Autodesk Inventor part; units mm, degrees
ref_plane "YZ Plane" through (0, 0, 0) normal (1, 0, 0) x (0, 1, 0)
ref_plane "XZ Plane" through (0, 0, 0) normal (0, 1, 0) x (-1, 0, 0)
ref_plane "XY Plane" through (0, 0, 0) normal (0, 0, 1) x (1, 0, 0)
sketch "Sketch1" plane through (0, 0, 0) normal (0, 1, 0) x (-1, 0, 0)
  circle A0 centre (0, 0) radius 56.769
  circle A1 centre (0, 0) radius 46.0756
  circle A2 centre (0, 0) radius 31.75
  dimension "d0" = 113.538
  dimension "d1" = 92.1512
  dimension "d2" = 63.5
extrude "Extrusion1" add sketch "Sketch1" along normal blind 17.272 contours A0 | A1 | A2
sketch "Sketch2" plane through (0, 17.272, 0) normal (0, 1, 0) x (1, 0, 0)
  circle A0 centre (0, 0) radius 46.0756
  circle A1 centre (-46.0756, 0) radius 4.0894
  dimension "d5" = 92.1512
  dimension "d6" = 8.1788
hole "Hole1" at (-46.0756, 17.272, 0) direction (0, -1, 0) diameter 8.4328 end through all
pattern_circular "Circular Pattern1" count 8 over 360 about axis through (0, 0, 0) along (0, 1, 0) of "Hole1"
sketch "Sketch4" plane through (0, 17.272, 0) normal (0, 1, 0) x (1, 0, 0)
  circle A0 centre (0, 0) radius 14.7993
hole "Hole2" at (0, 17.272, 0) direction (0, -1, 0) diameter 63.5 end through all
sketch "Sketch6" plane through (0, 0, 0) normal (0, 1, 0) x (-1, 0, 0)
  circle A0 centre (0, 0) radius 31.75
  circle A1 centre (0, 0) radius 19.05
extrude "Extrusion3" add sketch "Sketch6" along normal blind 17.272
sketch "Sketch7" plane through (0, 17.272, 0) normal (0, 1, 0) x (1, 0, 0)
  circle A0 centre (0, 0) radius 34.29
  circle A1 centre (0, 0) radius 31.75
  circle A2 centre (0, 0) radius 25.4
  circle A3 centre (0, 0) radius 27.94
  dimension "d35" = 68.58
  dimension "d36" = 63.5
  dimension "d37" = 50.8
  dimension "d38" = 55.88
extrude "Extrusion4" cut sketch "Sketch7" against normal blind 1.27 contours A0
sketch "Sketch9" plane through (0, 17.272, 0) normal (0, 1, 0) x (1, 0, 0)
  circle A0 centre (0, 0) radius 27.94
  circle A1 centre (0, 0) radius 31.75
  dimension "d45" = 55.88
  dimension "d46" = 63.5
extrude "Extrusion6" cut sketch "Sketch9" against normal blind 2.54
chamfer "Chamfer1" distance 0.254 angle 45 1 edges at (-46.0756, 17.272, -4.2164)
chamfer "Chamfer2" distance 0.254 angle 45 1 edges at (-46.0756, 0, -4.2164)
chamfer "Chamfer3" distance 0.762 angle 45 2 edges at (56.769, 17.272, 0) (56.769, 0, 0)
sketch "Sketch10" plane through (0, 17.272, 0) normal (0, 1, 0) x (1, 0, 0)
  circle A0 centre (32.5804, 32.5804) radius 4.2164
  circle A1 centre (46.0756, 0) radius 4.2164
  line L0 (32.5804, 32.5804) -> (46.0756, 0)
  line L1 (46.0756, 0) -> (39.328, 16.2902)
  circle A2 centre (-46.0756, 0) radius 4.4704
  circle A3 centre (-32.5804, -32.5804) radius 4.2164
  line L2 (-46.0756, 0) -> (-32.5804, -32.5804)
  line L3 (39.328, 16.2902) -> (-39.328, -16.2902)
  line L4 (-39.328, -16.2902) -> (52.9444, 21.9303)
  line L5 (-39.328, -16.2902) -> (60.5469, -16.2902) construction
  line L6 (52.9444, 21.9303) -> (-52.9809, -21.9454)
  line L7 (39.328, 16.2902) -> (39.6342, 15.551)
  line L8 (39.6342, 15.551) -> (39.0218, 17.0294)
  line L9 (39.0218, 17.0294) -> (52.0886, 22.4418)
  line L10 (39.0218, 17.0294) -> (53.1652, 17.0294) construction
  line L11 (52.0886, 22.4418) -> (31.2876, 13.8258)
  line L12 (39.6342, 15.551) -> (52.7487, 20.9832)
  circle A4 centre (0, 0) radius 56.769
  line L13 (39.6342, 15.551) -> (53.8292, 15.551) construction
  line L14 (52.7487, 20.9832) -> (52.7487, 20.9832)
  line L15 (52.7487, 20.9832) -> (31.9774, 12.3794)
  circle A5 centre (0, 0) radius 34.29
  line L16 (31.2876, 13.8258) -> (52.0886, 22.4418)
  line L17 (52.0886, 22.4418) -> (52.7487, 20.9832)
  line L18 (52.0886, 22.4418) -> (31.2876, 13.8258)
  point P0 (31.365, 13.8578)
  dimension "d58" = 22.5
  dimension "d59" = 0.8001
  dimension "d60" = 1.6002
  dimension "d61" = 22.5
  dimension "d62" = 22.5
extrude "Extrusion7" cut sketch "Sketch10" against normal blind 1.016 contours L9 L17 L4 L0 | L0 L3 A5 L11 | L4 L17 L12 L0 | L0 L15 A5 L3
sketch "Sketch11" plane through (0, 17.272, 0) normal (0, 1, 0) x (1, 0, 0)
  line L0 (31.365, 13.8578) -> (51.4323, 22.17)
  line L1 (52.0446, 20.6916) -> (31.9774, 12.3794)
  line L2 (51.4323, 22.17) -> (31.365, 13.8578)
  line L3 (31.365, 13.8578) -> (-52.6609, -20.9468)
  line L4 (52.0446, 20.6916) -> (31.9774, 12.3794)
  circle A0 centre (0, 0) radius 56.769
  line L5 (-52.1363, -22.4616) -> (31.9774, 12.3794)
  line L6 (-52.1363, -22.4616) -> (-52.6609, -20.9468)
  arc A1 (31.365, 13.8578) -> (31.9774, 12.3794) centre (0, 0) ccw
  circle A2 centre (0, 0) radius 34.29
  line L7 (-31.365, -13.8578) -> (-31.9774, -12.3794)
  point P0 (-31.365, -13.8578)
extrude "Extrusion8" cut sketch "Sketch11" against normal blind 1.016 contours A1 L5 L6 L3
sketch "Sketch13" plane through (0, 0, 0) normal (0, -1, 0) x (1, 0, 0)
  circle A0 centre (0, 0) radius 27.94
  circle A1 centre (0, 0) radius 31.75
  circle A2 centre (0, 0) radius 34.29
extrude "Extrusion9" cut sketch "Sketch13" against normal blind 2.54 contours A1
extrude "Extrusion10" cut sketch "Sketch13" against normal blind 1.27 contours A2
sketch "Sketch14" plane through (0, 0, 0) normal (0, -1, 0) x (1, 0, 0)
  line L0 (31.365, -13.8578) -> (52.0886, -22.4418)
  line L1 (52.7487, -20.9832) -> (31.9774, -12.3794)
  line L2 (-52.6609, 20.9468) -> (-31.9774, 12.3794)
  line L3 (-31.365, 13.8578) -> (-52.1363, 22.4616)
  line L4 (51.4323, -22.17) -> (52.0886, -22.4418)
  line L5 (52.0886, -22.4418) -> (31.365, -13.8578)
  arc A0 (52.7487, -20.9832) -> (-52.1363, 22.4616) centre (0, 0) ccw
  line L6 (31.9774, -12.3794) -> (52.7487, -20.9832)
  line L7 (52.7487, -20.9832) -> (52.0886, -22.4418)
  circle A1 centre (0, 0) radius 34.29
  line L8 (-31.9774, 12.3794) -> (-31.365, 13.8578)
  circle A2 centre (0, 0) radius 56.769
  line L9 (-52.1363, 22.4616) -> (-52.6609, 20.9468)
extrude "Extrusion11" cut sketch "Sketch14" against normal blind 1.016 contours A1 L1 L7 L0
extrude "Extrusion12" cut sketch "Sketch14" against normal blind 1.016 contours L2 L9 L3 A1
sketch "Sketch15" plane through (0, 0, 0) normal (0, 1, 0) x (-1, 0, 0)
  circle A0 centre (0, 0) radius 19.05
extrude "Extrusion13" add sketch "Sketch15" along normal blind 17.272
sketch "Sketch17" plane through (0, 0, 0) normal (0, -1, 0) x (1, 0, 0)
  circle A0 centre (0, 0) radius 27.94
hole "Hole4" at (0, 0, 0) direction (0, 1, 0) diameter 10.9982 end through all
sketch "Sketch18" plane through (0, 0, 0) normal (0, -1, 0) x (1, 0, 0)
  line L0 (0, 0) -> (-13.6144, 0)
  dimension "d103" = 13.6144
hole "Hole5" at (-13.6144, 0, 0) direction (0, 1, 0) diameter 4.9022 end through all
pattern_circular "Circular Pattern5" count 3 over 360 about axis through (0, 161.4933, 0) along (0, -1, 0) of "Hole5"
properties part number "4.5 flange"
Here's how the part is built. I have some questions about the finished solid (model axes, mm). A direction names the side the tool comes from. Coordinates: 2 decimals unless noted, no trailing zeros. Answer as CSV lines item,"result". Start each with the question number.
1. For pin 1 (6 mm diameter, centred on y = 3.5, z = 37, fed in from -X); pin 2 (1.5 mm diameter, centred on x = 45, y = 11.5, fed in from -Z); pin 3 (3 mm diameter, centred on x = -18.5, y = 15.5, fed in from +Z), each with a flat end and sliding along its axis, tell me the tip position at first contact or that it passes through.
2. We'd pull the mould along X, two halves only. Please class faces 4 (the flat face through (-14, 0, -32)), 5 (the flat face through (42, 1.016, -17)), 6 (the conical face through (20.35, 0.13, 52.32)): released by +X, released by -X, zero draft, split by the parting line, or undercut.
3. I need wall thicknesses on line 1 (X direction, y = 10.25, z = 0); line 2 (X direction, y = 4.75, z = -30) (3 decimals); line 3 (Z direction, x = 33.5, y = 4.5). Which ranges of each line are inside material? Lowest first, please. Write a range as [from, to].
4. On a 3-axis mill with a long thin cutter (end or side, diameter ignored), from which of +Z, -Z, +X, -X, +Y, -Y can I reach the whole of each face in a straight line? I mean faces 1 (the flat face through (-42.17, 16.77, 16.6)), 2 (the cylindrical face through (-11.22, 8.76, 0.53)), 3 (the flat face through (41.58, 0.5, -18.09)). Say none if no direction works.
5. I want a section at A-A, the plane z = 0. Count the separate pieces of the cut face and the enclosed holes in it, and give its area (3 significant figures).
Recorded:
1,pin 1,"stops at x = -45.46"
1,pin 2,"stops at z = -35.56"
1,pin 3,"stops at z = 54.16"
2,face 4,"zero draft"
2,face 5,"undercut"
2,face 6,"split by the parting line"
3,line 1,"x = [-56.77, -50.29], [-41.86, -16.07], [-11.16, -5.5], [5.5, 41.86], [50.29, 56.77]"
3,line 2,"x = [-48.195, -35.915], [-29.246, 29.246], [35.915, 48.195]"
3,line 3,"z = [-45.83, -36.7], [-28.47, 28.47], [36.7, 45.83]"
4,face 1,"+Y"
4,face 2,"+Y, -Y"
4,face 3,"-Y"
5,separate pieces,"5"
5,enclosed holes,"0"
5,area,"1,340 mm2"
